Could you check a few things on this model? Use its own coordinates, in mm. Coordinates: 2 decimals unless noted, no trailing zeros. Loops run counter-clockwise (first coordinate to the right, second up) from the corner with the lowest first, then second, coordinate; pieces in that order, holes last. Notation, with made-up numbers: M 59,51.25 L 96,51.25 A25 ccw 96,63.25 Z; hole C -4.5,-34.75 d11. An arc over 180 degrees is marked long. Write each question's results on one line, items separated by ' | '.
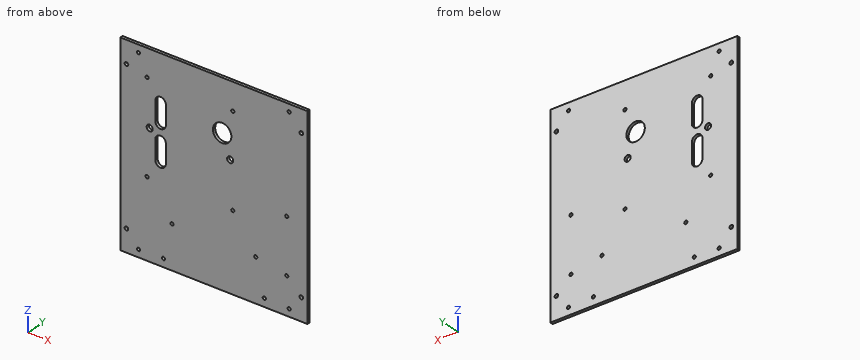
Autodesk Inventor part; units mm, degrees
ref_plane "YZ Plane" through (0, 0, 0) normal (1, 0, 0) x (0, 1, 0)
ref_plane "XZ Plane" through (0, 0, 0) normal (0, 1, 0) x (-1, 0, 0)
ref_plane "XY Plane" through (0, 0, 0) normal (0, 0, 1) x (1, 0, 0)
sketch "Sketch1" plane through (0, 0, 0) normal (0, 1, 0) x (-1, 0, 0)
  line L0 (98.0186, -101.2063) -> (-98.0186, -101.2063)
  line L1 (-98.0186, -101.2063) -> (-98.0186, 101.2063)
  line L2 (-98.0186, 101.2063) -> (98.0186, 101.2063)
  line L3 (98.0186, 101.2063) -> (98.0186, -101.2063)
  line L4 (98.0186, -101.2063) -> (-98.0186, 101.2063) construction
  line L5 (-98.0186, -101.2063) -> (98.0186, 101.2063) construction
  point P0 (0, 0)
  dimension "d0" = 196.0372
  dimension "d1" = 202.4126
extrude "Extrusion1" add sketch "Sketch1" along normal blind 3
sketch "Sketch2" plane through (0, 3, 0) normal (0, 1, 0) x (1, 0, 0)
  line L0 (98.0186, 101.2063) -> (-98.0186, 101.2063)
  line L1 (-98.0186, 101.2063) -> (-98.0186, -101.2063)
  line L2 (-98.0186, -101.2063) -> (98.0186, -101.2063)
  line L3 (98.0186, -101.2063) -> (98.0186, 101.2063)
  point P0 (0, 0)
  point P1 (-91.6686, 78.0923)
  point P2 (91.6686, 78.0923)
  point P3 (-91.6686, -78.0923)
  point P4 (91.6686, -78.0923)
  dimension "d4" = 23.114
  dimension "d5" = 23.114
  dimension "d6" = 6.35
  dimension "d7" = 6.35
hole "Hole1" at (-91.6686, 3, -78.0923) at (91.6686, 3, -78.0923) at (-91.6686, 3, 78.0923) at (91.6686, 3, 78.0923) direction (0, -1, 0) diameter 3.81 end through all
sketch "Sketch5" plane through (0, 3, 0) normal (0, 1, 0) x (1, 0, 0)
  line L0 (-98.0186, 101.2063) -> (-98.0186, -101.2063)
  line L1 (-98.0186, -101.2063) -> (98.0186, -101.2063)
  point P0 (0, 0)
  point P1 (-70.0786, -73.2663)
  point P2 (19.8374, -73.2663)
  point P3 (19.8374, 21.2217)
  point P4 (-70.0786, 21.2217)
  dimension "d44" = 27.94
  dimension "d45" = 27.94
  dimension "d46" = 89.916
  dimension "d47" = 94.488
hole "Hole4" at (-70.0786, 3, 73.2663) at (19.8374, 3, 73.2663) at (19.8374, 3, -21.2217) at (-70.0786, 3, -21.2217) direction (0, -1, 0) diameter 3.302 end through all
sketch "Sketch6" plane through (0, 3, 0) normal (0, 1, 0) x (1, 0, 0)
  circle A0 centre (-70.0786, -73.2663) radius 1.651
  circle A1 centre (19.8374, -73.2663) radius 1.651
  point P0 (0, 0)
  point P1 (-67.2846, -26.0223)
  point P2 (17.0434, -26.0223)
  dimension "d55" = 2.794
  dimension "d56" = 2.794
  dimension "d57" = 47.244
hole "Hole5" at (-67.2846, 3, 26.0223) at (17.0434, 3, 26.0223) direction (0, -1, 0) diameter 6.35 end through all
sketch "Sketch10" plane through (0, 3, 0) normal (0, 1, 0) x (1, 0, 0)
  line L0 (98.0186, 101.2063) -> (-98.0186, 101.2063)
  line L1 (98.0186, -101.2063) -> (98.0186, 101.2063)
  line L2 (0, 56.7563) -> (0, 92.8243)
  point P0 (0, 0)
  point P1 (-52.8574, 92.8243)
  point P2 (-43.9674, 56.7563)
  point P3 (52.8574, 92.8243)
  point P4 (43.9674, 56.7563)
  dimension "d91" = 52.8574
  dimension "d92" = 8.382
  dimension "d93" = 36.068
  dimension "d94" = 8.89
hole "Hole8" at (-52.8574, 3, -92.8243) at (-43.9674, 3, -56.7563) at (52.8574, 3, -92.8243) at (43.9674, 3, -56.7563) direction (0, -1, 0) diameter 3.302 end through all
sketch "Sketch11" plane through (0, 3, 0) normal (0, 1, 0) x (1, 0, 0)
  line L0 (98.0186, 101.2063) -> (-98.0186, 101.2063)
  line L1 (98.0186, -101.2063) -> (98.0186, 101.2063)
  point P0 (0, 0)
  point P1 (76.4286, 6.5913)
  point P2 (76.4286, 63.1063)
  dimension "d103" = 56.515
  dimension "d111" = 38.1
  dimension "d123" = 21.59
hole "Hole9" at (76.4286, 3, -6.5913) at (76.4286, 3, -63.1063) direction (0, -1, 0) diameter 3.302 end through all
sketch "Sketch12" plane through (0, 3, 0) normal (0, 1, 0) x (1, 0, 0)
  line L0 (98.0186, 101.2063) -> (-98.0186, 101.2063)
  line L1 (-98.0186, 101.2063) -> (-98.0186, -101.2063)
  line L2 (-98.0186, -101.2063) -> (98.0186, -101.2063)
  line L3 (98.0186, -101.2063) -> (98.0186, 101.2063)
  point P0 (0, 0)
  point P1 (-78.9686, -93.5863)
  point P2 (78.9686, -93.5863)
  point P3 (78.9686, 93.5863)
  point P4 (-78.9686, 93.5863)
  dimension "d112" = 7.62
  dimension "d113" = 19.05
  dimension "d114" = 7.62
  dimension "d115" = 19.05
hole "Hole10" at (-78.9686, 3, 93.5863) at (78.9686, 3, 93.5863) at (78.9686, 3, -93.5863) at (-78.9686, 3, -93.5863) direction (0, -1, 0) diameter 3.302 end through all
sketch "Sketch13" plane through (0, 3, 0) normal (0, 1, 0) x (1, 0, 0)
  line L0 (-55.88, 2.1463) -> (-55.88, -17.2847) construction
  line L1 (-61.4426, 2.1463) -> (-61.4426, -17.2847)
  line L2 (-50.3174, -17.2847) -> (-50.3174, 2.1463)
  arc A0 (-50.3174, 2.1463) -> (-61.4426, 2.1463) centre (-55.88, 2.1463) ccw
  arc A1 (-61.4426, -17.2847) -> (-50.3174, -17.2847) centre (-55.88, -17.2847) ccw
  circle A2 centre (-70.0786, 21.2217) radius 1.651
  line L3 (-55.88, -34.7599) -> (-55.88, -54.1909) construction
  line L4 (-61.4426, -34.7599) -> (-61.4426, -54.1909)
  line L5 (-50.3174, -54.1909) -> (-50.3174, -34.7599)
  arc A3 (-50.3174, -34.7599) -> (-61.4426, -34.7599) centre (-55.88, -34.7599) ccw
  arc A4 (-61.4426, -54.1909) -> (-50.3174, -54.1909) centre (-55.88, -54.1909) ccw
  point P0 (0, 0)
  point P1 (-55.88, -7.5692)
  point P2 (-55.88, -44.4754)
  dimension "d124" = 14.1986
  dimension "d125" = 11.1252
  dimension "d126" = 19.0754
  dimension "d127" = 19.431
  dimension "d128" = 19.431
  dimension "d129" = 11.1252
  dimension "d138" = 17.4752
extrude "Extrusion3" cut sketch "Sketch13" against normal through all contours A0 L2 A1 L1 | A3 L5 A4 L4
sketch "Sketch14" plane through (0, 3, 0) normal (0, 1, 0) x (1, 0, 0)
  circle A0 centre (8.6614, -48.4759) radius 9.652
  circle A1 centre (19.8374, -73.2663) radius 1.651
  point P0 (0, 0)
  dimension "d133" = 19.304
  dimension "d134" = 11.176
  dimension "d135" = 24.7904
extrude "Extrusion4" cut sketch "Sketch14" against normal through all contours A0
equation "\"d128\" = d127"
equation "\"d129\" = d125"
properties part number "SwarmieTopPlate"
(1) Imagine slicing it at C-C, the plane z = 46. List the corners of the cut face in (x, y) for me, and give its area (3 significant figures).
Reported:
outline: M -98.02,0 L -61.44,0 L -61.44,3 L -98.02,3 Z; M -50.32,0 L -0.67,0 L -0.67,3 L -50.32,3 Z; M 17.99,0 L 98.02,0 L 98.02,3 L 17.99,3 Z | area: 499 mm2
(2) Please list where these lines run through material, in increasing order: probe 1 along X at (y, z) = (0.4, -56.5); probe 2 along X at (y, z) = (2.95, 57); probe 3 along Z at (x, y) = (9.5, 1.75). Write a range as from..to.
Reported:
probe 1: x = -98.02..-45.6, -42.34..42.34, 45.6..98.02 | probe 2: x = -98.02..-60.68, -51.08..4.13, 13.19..98.02 | probe 3: z = -101.21..38.86, 58.09..101.21
(3) Imagine slicing it at B-B, the plane y = 2.05. State how many separate pieces and enclosed holes the cut face has, and give its area (3 significant figures).
Reported:
separate pieces: 1 | enclosed holes: 23 | area: 38,500 mm2
(4) Imagine slicing it at A-A, the plane z = 9.5. List the corners of the cut face in (x, y) for me.
Reported:
outline: M -98.02,0 L -61.44,0 L -61.44,3 L -98.02,3 Z; M -50.32,0 L 98.02,0 L 98.02,3 L -50.32,3 Z
